Input: part model. Units: mm. Frame: model coordinates. Coordinates: 2 decimals unless noted, no trailing zeros. Loops run counter-clockwise (first coordinate to the right, second up) from the corner with the lowest first, then second, coordinate; pieces in that order, holes last. Notation, with made-up numbers: (-18, 19.5) - (11, 19.5) arc R30 cw to (11, 42.5) - close; hole circle Ø2 at (-0.5, 25.5). An arc over 180 degrees is marked (long way). Use a Markdown table: item, result. Add a question column.
1. Section query C-C on z = 1. Return the cut outline in (x, y), then the cut area to 3 significant figures.
2. Section query B-B on y = 17. Return the cut outline in (x, z), then the cut area to 3 significant figures.
3. Section query A-A on x = 20. Return the cut outline in (y, z), then the cut area to 3 significant figures.
4. Ray query, L1, parallel to Y at x = 0, z = 1.4; L2, parallel to Y at x = 20, z = 1.6; L3, parallel to Y at x = 21.75, z = 1.45. Return the intervals inside material, ascending. Write a range as [from, to].
5. Contact query for flat-ended pins moving along their axis: P1, Ø0.6, axis at x = 17.5, z = 0.5, coming from the -Y side; P2, Ø5, axis at x = 19, y = 8.5, coming from the +Z side. Output: stop coordinate, or through.
6. Section query D-D on x = 0. Return the cut outline in (y, z).
```python
from build123d import *

# Parameters (mm, degrees)
SKETCH1_R           = 1.5
BOSS_EXTRUDE1_DEPTH = 2
FILLET1_R           = 2


with BuildPart() as part:
    # Sketch1 → Boss-Extrude1 (new body)
    with BuildSketch(Plane.XY):
        Polygon((-5, 12), (-5, -12), (5, -12), (5, 12), (25, 12), (25, 22), (-5, 22), align=None)
        with Locations((0, 9.5)):
            Circle(SKETCH1_R, mode=Mode.SUBTRACT)
        with Locations((0, -7.5)):
            Circle(SKETCH1_R, mode=Mode.SUBTRACT)
        with Locations((5, 17)):
            Circle(SKETCH1_R, mode=Mode.SUBTRACT)
        with Locations((20, 17)):
            Circle(SKETCH1_R, mode=Mode.SUBTRACT)
    extrude(amount=BOSS_EXTRUDE1_DEPTH)

    # Fillet1
    fillet1_edges = [part.edges().sort_by_distance(p)[0] for p in [
        (5, -12, 1),
        (-5, -12, 1),
        (-5, 22, 1),
        (25, 22, 1),
        (25, 12, 1),
    ]]
    fillet(fillet1_edges, radius=FILLET1_R)


solid = part.part
```
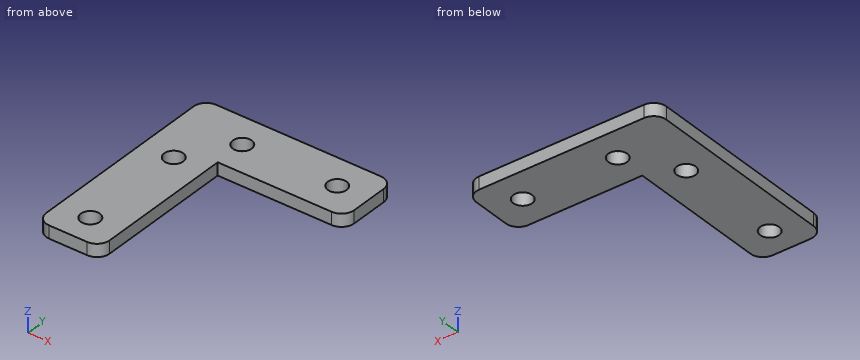
Resolved:
| question | item | result |
|---|---|---|
| 1 | outline | (-5, -10) arc R2 ccw to (-3, -12) - (3, -12) arc R2 ccw to (5, -10) - (5, 12) - (23, 12) arc R2 ccw to (25, 14) - (25, 20) arc R2 ccw to (23, 22) - (-3, 22) arc R2 ccw to (-5, 20) - close; hole circle Ø3 at (0, -7.5); hole circle Ø3 at (0, 9.5); hole circle Ø3 at (5, 17); hole circle Ø3 at (20, 17) |
| 1 | area | 507 mm² |
| 2 | outline | (-5, 0) - (3.5, 0) - (3.5, 2) - (-5, 2) - close; (6.5, 0) - (18.5, 0) - (18.5, 2) - (6.5, 2) - close; (21.5, 0) - (25, 0) - (25, 2) - (21.5, 2) - close |
| 2 | area | 48.0 mm² |
| 3 | outline | (12, 0) - (15.5, 0) - (15.5, 2) - (12, 2) - close; (18.5, 0) - (22, 0) - (22, 2) - (18.5, 2) - close |
| 3 | area | 14.0 mm² |
| 4 | L1 | [-12, -9], [-6, 8], [11, 22] |
| 4 | L2 | [12, 15.5], [18.5, 22] |
| 4 | L3 | [12, 22] |
| 5 | P1 | y = 12 |
| 5 | P2 | through |
| 6 | outline | (-12, 0) - (-9, 0) - (-9, 2) - (-12, 2) - close; (-6, 0) - (8, 0) - (8, 2) - (-6, 2) - close; (11, 0) - (22, 0) - (22, 2) - (11, 2) - close |
